from build123d import *

# Parameters (mm, degrees)
SKETCH1_R           = 2.54
BOSS_EXTRUDE1_DEPTH = 3.81
SKETCH2_R           = 3.302
CUT_EXTRUDE3_DEPTH  = 0.635


with BuildPart() as part:
    # Sketch1 → Boss-Extrude1 (new body)
    with BuildSketch(Plane.XY):
        with BuildLine():
            ThreePointArc((7.874, -3.81), (11.684, 0), (7.874, 3.81))
            Line((7.874, 3.81), (-7.874, 3.81))
            ThreePointArc((-7.874, 3.81), (-11.684, 0), (-7.874, -3.81))
            Line((-7.874, -3.81), (7.874, -3.81))
        make_face()
        with BuildLine():
            ThreePointArc((-2.95121331, 3.302), (-2.484585514, 2.994804631), (-2.582311646, 2.44475))
            ThreePointArc((-2.582311646, 2.44475), (-3.556, 0), (-2.582311646, -2.44475))
            ThreePointArc((-2.582311646, -2.44475), (-2.484585514, -2.994804631), (-2.95121331, -3.302))
            Line((-2.95121331, -3.302), (-4.92278669, -3.302))
            ThreePointArc((-4.92278669, -3.302), (-5.389414486, -2.994804631), (-5.291688354, -2.44475))
            ThreePointArc((-5.291688354, -2.44475), (-4.318, 0), (-5.291688354, 2.44475))
            ThreePointArc((-5.291688354, 2.44475), (-5.389414486, 2.994804631), (-4.92278669, 3.302))
            Line((-4.92278669, 3.302), (-2.95121331, 3.302))
        make_face(mode=Mode.SUBTRACT)
        Circle(SKETCH1_R, mode=Mode.SUBTRACT)
        with BuildLine():
            Line((4.92278669, -3.302), (2.95121331, -3.302))
            ThreePointArc((2.95121331, -3.302), (2.484585514, -2.994804631), (2.582311646, -2.44475))
            ThreePointArc((2.582311646, -2.44475), (3.556, 0), (2.582311646, 2.44475))
            ThreePointArc((2.582311646, 2.44475), (2.484585514, 2.994804631), (2.95121331, 3.302))
            Line((2.95121331, 3.302), (4.92278669, 3.302))
            ThreePointArc((4.92278669, 3.302), (5.389414486, 2.994804631), (5.291688354, 2.44475))
            ThreePointArc((5.291688354, 2.44475), (4.731418896, 1.664127401), (4.40060224, 0.762))
            Line((4.40060224, 0.762), (7.112, 0.762))
            Line((7.112, 0.762), (7.112, 1.524))
            ThreePointArc((7.112, 1.524), (7.874, 2.286), (8.636, 1.524))
            Line((8.636, 1.524), (8.636, 0.762))
            Line((8.636, 0.762), (9.398, 0.762))
            ThreePointArc((9.398, 0.762), (10.16, 0), (9.398, -0.762))
            Line((9.398, -0.762), (8.636, -0.762))
            Line((8.636, -0.762), (8.636, -1.524))
            ThreePointArc((8.636, -1.524), (7.874, -2.286), (7.112, -1.524))
            Line((7.112, -1.524), (7.112, -0.762))
            Line((7.112, -0.762), (4.40060224, -0.762))
            ThreePointArc((4.40060224, -0.762), (4.731418896, -1.664127401), (5.291688354, -2.44475))
            ThreePointArc((5.291688354, -2.44475), (5.389414486, -2.994804631), (4.92278669, -3.302))
        make_face(mode=Mode.SUBTRACT)
        with Locations((-7.874, 0)):
            Circle(SKETCH1_R, mode=Mode.SUBTRACT)
    extrude(amount=BOSS_EXTRUDE1_DEPTH)

    # Sketch2 → Cut-Extrude3 (cut)
    with BuildSketch(Plane.XY):
        Circle(SKETCH2_R)
        with Locations((-7.874, 0)):
            Circle(SKETCH2_R)
    extrude(amount=CUT_EXTRUDE3_DEPTH, mode=Mode.SUBTRACT)

    # Mirror1: part across face


with BuildPart() as part_1:
    add(part.part)
    add(part.part.mirror(Plane(origin=(0.730328886, 0, 3.81), x_dir=(1, 0, 0), z_dir=(0, 0, 1))))


solid = part_1.part
Read the model definition and answer for the solid it produces. Units are mm, in the model's axes. A direction names the side the tool comes from. Give positions to 0.01 mm unless a question says otherwise; leave off trailing zeros. Write each loop counter-clockwise with the first axis right and the second up, starting at its lowest first coordinate (ties: lowest second). Pieces come first, ordered by that corner, then holes. Notation, with made-up numbers: (8.25, 57) -> (30.25, 57) arc R19 ccw to (30.25, 77) -> close; hole circle Ø7 at (81, 82). An arc over 180 degrees is marked (long way). Answer as a JSON object with one key per item and string values. Group by question number.
1) Find section D-D (x = 0). Write down the section's boundary in (y, z) (3 decimals), and give its area (3 significant figures).
2) The mould has two halves that part along Y. Classify faces 5 (the flat face through (-4, 3.302, 4)), 6 (the flat face through (2, -2, 6.985)), 7 (the flat face through (0, -3.81, 4)), 8 (the flat face through (0, 3.81, 4)): +Y half, -Y half, draft (parallel to the pull), parting line (faces both ways), or undercut.
3) Each of these flat-tipped pins is pushed along its axis until it touches: P1, Ø3, axis at x = -9, z = 1, coming from the +Y side; P2, Ø0.6, axis at y = 1.5, z = 3, coming from the +X side; P3, Ø0.8, axis at y = -1, z = 4.5, coming from the +X side. Where does it stop, or does it pass through?
4) Find section B-B (z = 5). Count the separate pieces of the cut face and the enclosed holes in it, and give its area (3 significant figures).
5) Consider L1, parallel to X at y = 0, z = 4.8; L2, parallel to X at y = -1.25, z = 6.25; L3, parallel to X at y = -0.5, z = 4.5. Determine where each line is inside the solid, lowest interval first. Write a range as from..to.
6) A tool of negligible diameter and unlimited length cuts with its end or side. For faces 1 (the cylindrical face through (11.683, -0.084, 3.863)), 2 (the cylindrical face through (-3.556, 0.038, 3.863)), 3 (the cylindrical face through (3.05, -1.26, 0.31)), 4 (the cylindrical face through (3.05, -1.26, 7.31)), from which of +Z, -Z, +X, -X, +Y, -Y can it reach the whole face along a straight path? Write none if from no direction.
7) Find section A-A (x = 6.5). Write down the section's boundary in (y, z), and give its area (3 significant figures).
Values follow:
{
 "1": {"outline": "(-3.81, 0) -> (-3.302, 0) -> (-3.302, 0.635) -> (-2.54, 0.635) -> (-2.54, 6.985) -> (-3.302, 6.985) -> (-3.302, 7.62) -> (-3.81, 7.62) -> close; (2.54, 0.635) -> (3.302, 0.635) -> (3.302, 0) -> (3.81, 0) -> (3.81, 7.62) -> (3.302, 7.62) -> (3.302, 6.985) -> (2.54, 6.985) -> close", "area": "17.4 mm2"},
 "2": {"face 5": "undercut", "face 6": "undercut", "face 7": "-Y half", "face 8": "+Y half"},
 "3": {"P1": "stops at y = 3.81", "P2": "stops at x = 11.49", "P3": "stops at x = 11.64"},
 "4": {"separate pieces": "1", "enclosed holes": "4", "area": "89.2 mm2"},
 "5": {"L1": "x = -11.68..-10.41, -5.33..-4.32, -3.56..-2.54, 2.54..3.56, 10.16..11.68", "L2": "x = -11.47..-10.09, -5.66..-4.54, -3.33..-2.21, 2.21..3.33, 4.54..7.11, 8.64..11.47", "L3": "x = -11.65..-10.36, -5.38..-4.35, -3.52..-2.49, 2.49..3.52, 9.97..11.65"},
 "6": {"face 1": "+Z, -Z, +X", "face 2": "+Z, -Z", "face 3": "-Z", "face 4": "+Z"},
 "7": {"outline": "(-3.81, 0) -> (-0.76, 0) -> (-0.76, 7.62) -> (-3.81, 7.62) -> close; (0.76, 0) -> (3.81, 0) -> (3.81, 7.62) -> (0.76, 7.62) -> close", "area": "46.5 mm2"}
}
